The drawing under review shows one solid part. Ordinate dimensions are in mm from its lowest x, y, z. A direction names the side the tool comes from. Coordinates: 2 decimals unless noted, no trailing zeros. Write each loop counter-clockwise with the first axis right and the second up, starting at its lowest first coordinate (ties: lowest second). Pieces come first, ordered by that corner, then holes.
Q1. Machinability: for the marked faces 4 and 5, which of the approach directions +Z, -Z, +X, -X, +Y, -Y give a long, thin tool a straight path to every point of the face, cutting with its end or side? Answer none if there is none.
Q2. Add section A-A, the plane x = 30. Give the boundary of the cut face in (y, z), plus the area to 3 significant figures.
Q3. Add section C-C, the plane z = 7.5. Give the boundary of the cut face in (x, y).
Q4. Clearance check with flat-ended pins moving along their axes: pin 1 Ø8 at (x, z) = (32, 4.5) entering from +Y; pin 2 Ø2 at (y, z) = (26.5, 10.5) entering from -X; pin 3 Ø4 at (x, z) = (34.5, 11.5) entering from -Y. State where each tip first meets the part, or that it passes through.
Q5. Add section D-D, the plane y = 12. Give the boundary of the cut face in (x, z), plus the area to 3 significant figures.
Q6. Add section B-B, the plane y = 30. Give the boundary of the cut face in (x, z), plus the area to 3 significant figures.
Q7. The part is to be moulded in two halves that separate along Y. For the marked faces 1, 2 and 3, say which applies: +Y half, -Y half, draft (parallel to the pull), parting line (faces both ways), or undercut.
Q8. To check wall thickness, follow probe 1 along Z at (x, y) = (33, 29); probe 2 along Z at (x, y) = (11, 20); probe 3 along X at (y, z) = (38, 26.75) (1 decimal). State the ranges of each line that lie inside material, in increasing order.
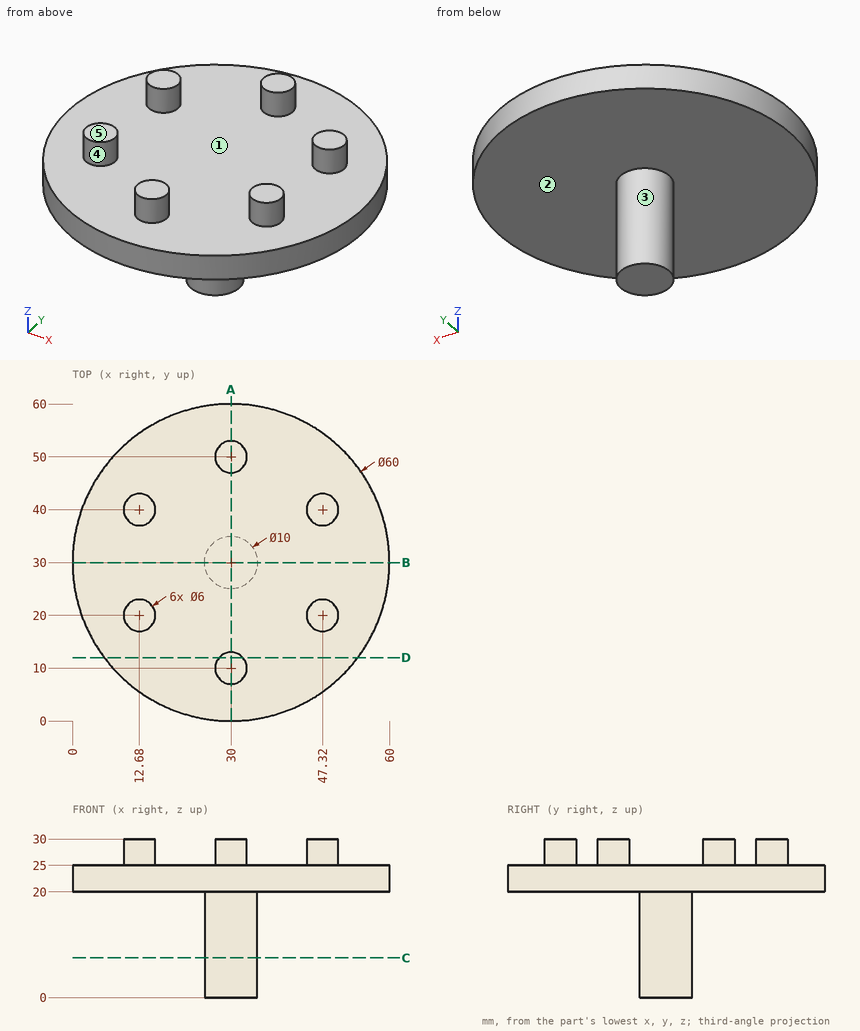
Here are the results:
1. face 4: +Z
1. face 5: +Z, +X, -X, +Y, -Y
2. outline: (0, 20) - (25, 20) - (25, 0) - (35, 0) - (35, 20) - (60, 20) - (60, 25) - (53, 25) - (53, 30) - (47, 30) - (47, 25) - (13, 25) - (13, 30) - (7, 30) - (7, 25) - (0, 25) - close
2. area: 560 mm2
3. outline: circle Ø10 at (30, 30)
4. pin 1: stops at y = 35
4. pin 2: stops at x = 25.67
4. pin 3: stops at y = 25.67
5. outline: (6, 20) - (54, 20) - (54, 25) - (32.24, 25) - (32.24, 30) - (27.76, 30) - (27.76, 25) - (6, 25) - close
5. area: 262 mm2
6. outline: (0, 20) - (25, 20) - (25, 0) - (35, 0) - (35, 20) - (60, 20) - (60, 25) - (0, 25) - close
6. area: 500 mm2
7. face 1: undercut
7. face 2: draft
7. face 3: parting line
8. probe 1: z = 0 to 25
8. probe 2: z = 20 to 30
8. probe 3: x = 10.4 to 14.9, 45.1 to 49.6
